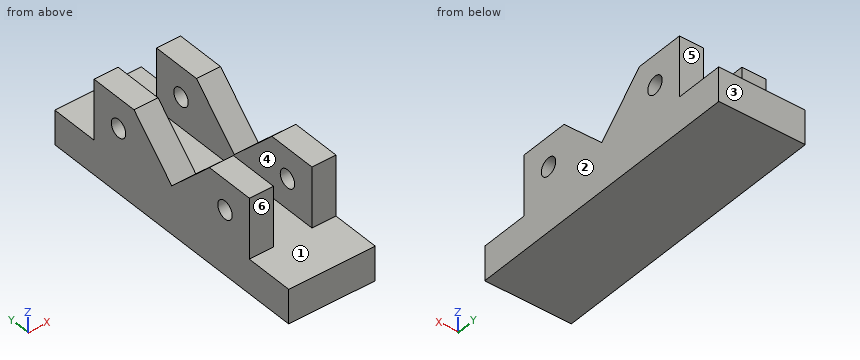
from build123d import *

# Parameters (mm, degrees)
SKETCH_W        = 63
SKETCH_H        = 211
PAD_DEPTH       = 25
SKETCH001_W     = 17.5
SKETCH001_H     = 140
PAD001_DEPTH    = 44
POCKET_DEPTH    = 63
SKETCH003_R     = 6.5
POCKET001_DEPTH = 63


with BuildPart() as part:
    # Sketch → Pad (new body)
    with BuildSketch(Plane.XY):
        with Locations((31.5, 105.5)):
            Rectangle(SKETCH_W, SKETCH_H)
    extrude(amount=PAD_DEPTH)

    # Sketch001 (on Face6 of Pad) → Pad001 (join)
    with BuildSketch(Plane.XY.offset(25)):
        with Locations((8.75, 105.5)):
            Rectangle(SKETCH001_W, SKETCH001_H)
        with Locations((54.25, 105.5)):
            Rectangle(SKETCH001_W, SKETCH001_H)
    extrude(amount=PAD001_DEPTH)

    # Sketch002 (on Face8 of Pad001) → Pocket (cut)
    with BuildSketch(Plane.YZ.offset(63)):
        Polygon((71.5, 69), (105.5, 35), (139.5, 69), align=None)
    extrude(amount=-POCKET_DEPTH, mode=Mode.SUBTRACT)

    # Sketch003 (on Face8 of Pocket) → Pocket001 (cut)
    with BuildSketch(Plane.YZ.offset(63)):
        with Locations((57.5, 47)):
            Circle(SKETCH003_R)
        with Locations((153.5, 47)):
            Circle(SKETCH003_R)
    extrude(amount=-POCKET001_DEPTH, mode=Mode.SUBTRACT)


solid = part.part
Here's how the part is built. I have some questions about the finished solid (model axes, mm). Face numbers are marked on the shaded views. A direction names the side the tool comes from. Give positions to 0.01 mm unless a question says otherwise; leave off trailing zeros. Order: outer loops, then holes, each group sorted by start corner. A loop starts at its lowest first (then second) coordinate and runs counter-clockwise, first axis right, second up. Notation, with made-up numbers: (47.5, 87) -> (106.5, 87) arc R25 cw to (106.5, 101) -> close; hole circle Ø1 at (33, 78.25). An arc over 180 degrees is marked (long way). Use a Markdown table: item, result. Add a question column.
Item 1: If we mould it in two halves opening along X, with no side actions, what happens to the marked faces 1, 2 and 3? For each: pulls with the +X half, pulls with the -X half, needs draft (parallel to the pull), parting line crosses it, or undercut.
Item 2: Imagine slicing it at D-D on y = 114. Please give me the cut outline in (x, z).
Item 3: Imagine slicing it at B-B on y = 60. Please give me the cut outline in (x, z).
Item 4: Imagine slicing it at C-C on x = 7. Please give me the cut outline in (y, z).
Item 5: For the marked faces 4, 5 and 6, which set-ups out of +Z, -Z, +X, -X, +Y, -Y let a thin tool reach every point of the face, with its end or its side?
Item 6: I need wall thicknesses on line 1 (X direction, y = 94, z = 38); line 2 (Z direction, x = 50.25, y = 57.5); line 3 (Y direction, x = 15, z = 47.5). Which ranges of each line are inside material? Lowest first, please.
Item 7: Will these pins go through, and if not, where does the flat tip stop? pin 1 (19 mm diameter, centred on x = 5, z = 45, fed in from -Y); pin 2 (5 mm diameter, centred on x = 10, z = 46.5, fed in from +Y); pin 3 (5 mm diameter, centred on x = 8, y = 102.5, fed in from +Z).
Item 8: Imagine slicing it at A-A on z = 47. Give the number of separate pieces and of enclosed holes in the cut face, plus the area to 3 significant figures.
Data:
| question | item | result |
|---|---|---|
| 1 | face 1 | undercut |
| 1 | face 2 | pulls with the +X half |
| 1 | face 3 | needs draft |
| 2 | outline | (0, 0) -> (63, 0) -> (63, 43.5) -> (45.5, 43.5) -> (45.5, 25) -> (17.5, 25) -> (17.5, 43.5) -> (0, 43.5) -> close |
| 3 | outline | (0, 0) -> (63, 0) -> (63, 41) -> (45.5, 41) -> (45.5, 25) -> (17.5, 25) -> (17.5, 41) -> (0, 41) -> close; (0, 53) -> (17.5, 53) -> (17.5, 69) -> (0, 69) -> close; (45.5, 53) -> (63, 53) -> (63, 69) -> (45.5, 69) -> close |
| 4 | outline | (0, 0) -> (211, 0) -> (211, 25) -> (175.5, 25) -> (175.5, 69) -> (139.5, 69) -> (105.5, 35) -> (71.5, 69) -> (35.5, 69) -> (35.5, 25) -> (0, 25) -> close; hole circle Ø13 at (57.5, 47); hole circle Ø13 at (153.5, 47) |
| 5 | face 4 | +Z, +Y, -Y |
| 5 | face 5 | +Z, +X, -X, +Y |
| 5 | face 6 | +Z, +X, -X, -Y |
| 6 | line 1 | x = 0 to 17.5, 45.5 to 63 |
| 6 | line 2 | z = 0 to 40.5, 53.5 to 69 |
| 6 | line 3 | y = 35.5 to 51.02, 63.98 to 93, 118 to 147.02, 159.98 to 175.5 |
| 7 | pin 1 | stops at y = 35.5 |
| 7 | pin 2 | stops at y = 175.5 |
| 7 | pin 3 | stops at z = 40.5 |
| 8 | separate pieces | 8 |
| 8 | enclosed holes | 0 |
| 8 | area | 3,150 mm² |
